Work out the finished part from the listing and answer in its coordinate system (mm). Face numbers are marked on the shaded views. A direction names the side the tool comes from. Coordinates: 2 decimals unless noted, no trailing zeros. Loops run counter-clockwise (first coordinate to the right, second up) from the corner with the lowest first, then second, coordinate; pieces in that order, holes last. Notation, with made-up numbers: M 12.25,53 L 52.25,53 A11 cw 52.25,67 Z; hole C 61.5,10.25 d1. An arc over 180 degrees is marked long. Write each question's results on one line, items separated by ' | '.
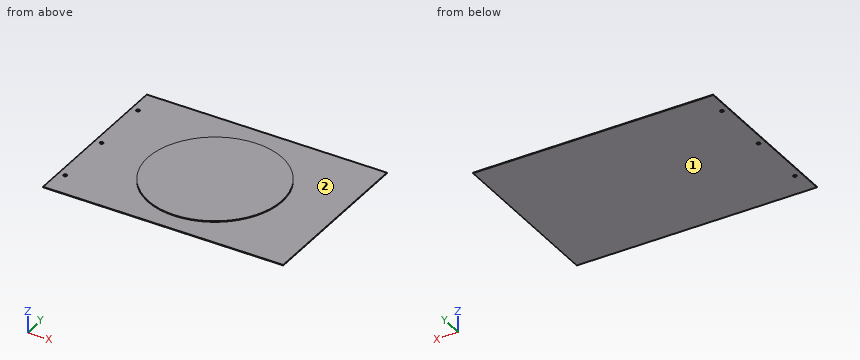
```python
from build123d import *

# Parameters (mm, degrees)
F0_W     = 430
F0_H     = 307
F0_R     = 3
F1_DEPTH = 1
F2_DEPTH = 2


with BuildPart() as f1:
    # F0 (on Top) → F1 (new body)
    with BuildSketch(Plane.XY):
        Rectangle(F0_W, F0_H)
        with Locations((-203, -108)):
            Circle(F0_R, mode=Mode.SUBTRACT)
        with Locations((-203, 0)):
            Circle(F0_R, mode=Mode.SUBTRACT)
        with Locations((-203, 108)):
            Circle(F0_R, mode=Mode.SUBTRACT)
        with BuildLine():
            ThreePointArc((0, 120), (84.852814, 84.852814), (120, 0))
            ThreePointArc((120, 0), (84.852814, -84.852814), (0, -120))
            ThreePointArc((0, -120), (-84.852814, -84.852814), (-120, 0))
            ThreePointArc((-120, 0), (-84.852814, 84.852814), (0, 120))
        make_face(mode=Mode.SUBTRACT)
    extrude(amount=F1_DEPTH)

    # F0 (on Top) → F2 (join)
    with BuildSketch(Plane.XY):
        with BuildLine():
            Line((0, 0), (0, 120))
            ThreePointArc((0, 120), (-84.852814, 84.852814), (-120, 0))
            Line((-120, 0), (0, 0))
        make_face()
        with BuildLine():
            Line((0, 0), (120, 0))
            ThreePointArc((120, 0), (84.852814, 84.852814), (0, 120))
            Line((0, 120), (0, 0))
        make_face()
        with BuildLine():
            ThreePointArc((0, -120), (84.852814, -84.852814), (120, 0))
            Line((120, 0), (0, 0))
            Line((0, 0), (0, -120))
        make_face()
        with BuildLine():
            ThreePointArc((-120, 0), (-84.852814, -84.852814), (0, -120))
            Line((0, -120), (0, 0))
            Line((0, 0), (-120, 0))
        make_face()
    extrude(amount=F2_DEPTH)


solid = f1.part
```
1) Straight lines are drawn through the part: probe 1 along Y at (x, z) = (-203, 0.4); probe 2 along Z at (x, y) = (-73, 122); probe 3 along X at (y, z) = (26, 1.55). For each, find the intervals that lie inside material, in ascending order. Write a range as [from, to].
Check result:
probe 1: [-153.5, -111], [-105, -3], [3, 105], [111, 153.5] | probe 2: [0, 1] | probe 3: [-117.15, 117.15]
2) Find section D-D, the plane x = -9. Give the vertices of the cut face in (y, z).
Check result:
outline: M -153.5,0 L 153.5,0 L 153.5,1 L 119.66,1 L 119.66,2 L -119.66,2 L -119.66,1 L -153.5,1 Z
3) Which of the six approach directions +Z, -Z, +X, -X, +Y, -Y give full straight-line access (tool end or side, diameter ignored) to the marked faces 1 and 2?
Check result:
face 1: -Z, +X, -X, +Y, -Y | face 2: +Z
4) Find section B-B, the plane x = 133. Give the vertices of the cut face in (y, z).
Check result:
outline: M -153.5,0 L 153.5,0 L 153.5,1 L -153.5,1 Z
5) Find section A-A, the plane y = -41.5. Give the vertices of the cut face in (x, z).
Check result:
outline: M -215,0 L 215,0 L 215,1 L 112.6,1 L 112.6,2 L -112.6,2 L -112.6,1 L -215,1 Z
6) Find section C-C, the plane z = 1.6. Give the vertices of the cut face in (x, y), and give its area (3 significant figures).
Check result:
outline: M -120,0 A120 ccw 0,-120 A120 ccw 120,0 A120 ccw 0,120 A120 ccw Z | area: 45,200 mm^2
7) Given pin 1 Ø9.5 at (x, y) = (-203, 108) entering from -Z; pin 2 Ø5 at (x, y) = (-109, -65) entering from +Z, each flat-ended and moving along its own axis, determine where each tip first touches the part or whether it passes through.
Check result:
pin 1: z = 0 | pin 2: z = 1
